Print and shaded views of the part. All mm, measured from the part's lowest x, y and z. A direction names the side the tool comes from. Round coordinates to 2 decimals unless told otherwise and drop trailing zeros. Write each loop counter-clockwise with the first axis right and the second up, starting at its lowest first coordinate (ties: lowest second). Pieces come first, ordered by that corner, then holes. Notation, with made-up numbers: (58, -8) - (63, -8) arc R4 cw to (63, -1) - close; hole circle Ø5 at (6.25, 41). An arc over 180 degrees is marked (long way). Answer as a JSON object with one key per item and string values. Group by question number.
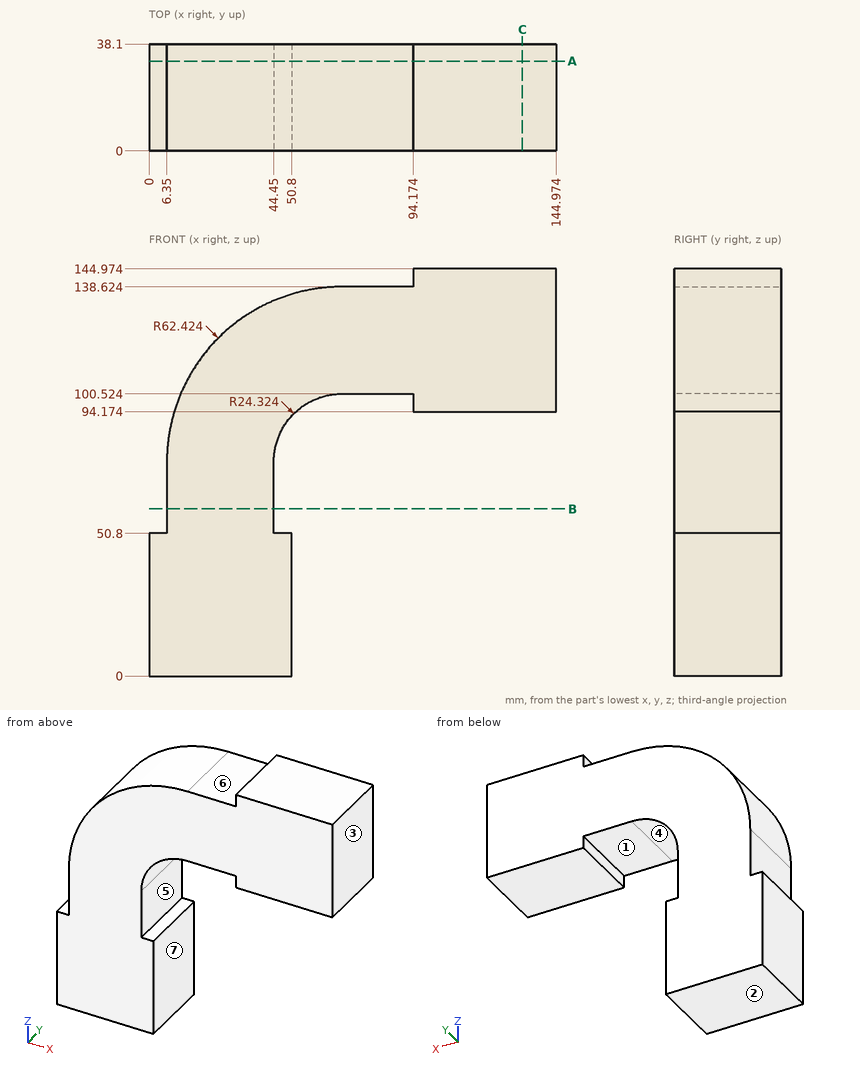
(1) Drill centre lines: line 1 (X direction, y = 15.5, z = 52.5); line 2 (X direction, y = 35.5, z = 38.5); line 3 (Z direction, x = 101.5, y = 23.5). Where is each one in solid material? Low to high. Write a range as from..to.
(2) Flat gauge pins, fed straight in: pin 1 (3 mm diameter, centred on x = 48, y = 13, fed in from +Z); pin 2 (1.5 mm diameter, centred on x = 31.5, y = 32, fed in from +Z); pin 3 (5 mm diameter, centred on x = 3, y = 19.5, fed in from +Z). Where does each tip first touch, or does it go through?
(3) Slice it at A-A (y = 32). Write the cut outline in (x, z), then the cut area to 3 significant figures.
(4) Slice it at B-B (z = 59.5). Write the cut outline in (x, y), then the cut area to 3 significant figures.
(5) 3-axis set-ups, long thin cutter, end or side, ignore diameter. For the marked faces 4, 5, 6 and 7: which of +Z, -Z, +X, -X, +Y, -Y reach the whole face in a straight line?
(6) Slice it at C-C (x = 133). Write the cut outline in (y, z), then the cut area to 3 significant figures.
(7) Pull direction X, two halves, no side cores. Call the marked faces 1, 2 and 3: pulls with the +X half, pulls with the -X half, needs draft (parallel to the pull), parting line crosses it, or undercut.
Answer:
{
 "1": {"line 1": "6.35..44.45", "line 2": "0..50.8", "line 3": "94.17..144.97"},
 "2": {"pin 1": "z = 135.57", "pin 2": "z = 126.82", "pin 3": "z = 50.8"},
 "3": {"outline": "(0, 0) - (50.8, 0) - (50.8, 50.8) - (44.45, 50.8) - (44.45, 76.2) arc R24.32 cw to (68.77, 100.52) - (94.17, 100.52) - (94.17, 94.17) - (144.97, 94.17) - (144.97, 144.97) - (94.17, 144.97) - (94.17, 138.62) - (68.77, 138.62) arc R62.42 ccw to (6.35, 76.2) - (6.35, 50.8) - (0, 50.8) - close", "area": "9,690 mm²"},
 "4": {"outline": "(6.35, 0) - (44.45, 0) - (44.45, 38.1) - (6.35, 38.1) - close", "area": "1,450 mm²"},
 "5": {"face 4": "+Y, -Y", "face 5": "+X, +Y, -Y", "face 6": "+Z, -X, +Y, -Y", "face 7": "-Z, +X, +Y, -Y"},
 "6": {"outline": "(0, 94.17) - (38.1, 94.17) - (38.1, 144.97) - (0, 144.97) - close", "area": "1,940 mm²"},
 "7": {"face 1": "undercut", "face 2": "needs draft", "face 3": "pulls with the +X half"}
}
